```python
from build123d import *

# Parameters (mm, degrees)
SKETCH_2_R           = 9.5
EXTRUDE_1_DEPTH      = 40
SKETCH_3_W           = 6
SKETCH_3_H           = 6
EXTRUDE_2_DEPTH      = 0.1
EXTRUDE_2_DEPTH_BACK = 25
CHAMFER_1_SIZE       = 1
SKETCH_4_R           = 100
EXTRUDE_3_DEPTH      = 10
SKETCH_5_R           = 60
SKETCH_5_R_2         = 15
CUT_EXTRUDE_1_DEPTH  = 4
SKETCH_7_R           = 65
SKETCH_7_R_2         = 60
EXTRUDE_4_DEPTH      = 3.5
CHAMFER_2_SIZE       = 1
SKETCH_8_R           = 6
CUT_EXTRUDE_2_DEPTH  = 11
CHAMFER_3_SIZE       = 1
SKETCH_9_R           = 58
EXTRUDE_5_DEPTH      = 38
SKETCH_10_R          = 63
EXTRUDE_6_DEPTH      = 123
SKETCH_11_R          = 65
EXTRUDE_7_DEPTH      = 61.5
CHAMFER_4_SIZE       = 25
EXTRUDE_8_DEPTH      = 104
CUT_EXTRUDE_3_REACH  = 173
SKETCH_13_R          = 3.5
SKETCH_14_W          = 60
SKETCH_14_H          = 60
EXTRUDE_9_DEPTH      = 117
SKETCH_15_R          = 15
EXTRUDE_10_DEPTH     = 68
CHAMFER_5_SIZE       = 1
SKETCH_17_R          = 7
SKETCH_18_R          = 9
EXTRUDE_11_DEPTH     = 8
EXTRUDE_12_DEPTH     = 10
SKETCH_20_R          = 6
CUT_EXTRUDE_4_DEPTH  = 10


with BuildPart() as part:
    # Эскиз2 → Вытянуть1 (new body)
    with BuildSketch(Plane.XY):
        Circle(SKETCH_2_R)
    extrude(amount=EXTRUDE_1_DEPTH)

    # Эскиз3 → Вытянуть2 (add, two sides)
    with BuildSketch(Plane(origin=(0, 0, 0), x_dir=(-1, 0, 0), z_dir=(0, 0, -1))) as extrude_2_sk:
        with Locations((0, 9)):
            Rectangle(SKETCH_3_W, SKETCH_3_H)
    extrude(amount=EXTRUDE_2_DEPTH)
    extrude(extrude_2_sk.sketch, amount=-EXTRUDE_2_DEPTH_BACK)

    # Фаска1
    chamfer_1_edges = [part.edges().sort_by_distance(p)[0] for p in [
        (-5.556527693, -7.705517504, 0),
    ]]
    chamfer(chamfer_1_edges, length=CHAMFER_1_SIZE)

    # Эскиз4 → Вытянуть3 (add)
    with BuildSketch(Plane.XY.offset(40)):
        Circle(SKETCH_4_R)
    extrude(amount=EXTRUDE_3_DEPTH)

    # Эскиз5 → Вырез-Вытянуть1 (cut)
    with BuildSketch(Plane(origin=(0, 0, 40), x_dir=(-1, 0, 0), z_dir=(0, 0, -1))):
        Circle(SKETCH_5_R)
        Circle(SKETCH_5_R_2, mode=Mode.SUBTRACT)
    extrude(amount=-CUT_EXTRUDE_1_DEPTH, mode=Mode.SUBTRACT)

    # Эскиз7 → Вытянуть4 (add)
    with BuildSketch(Plane(origin=(0, 0, 40), x_dir=(-1, 0, 0), z_dir=(0, 0, -1))):
        with Locations(Location((0, 0, 0), (0, 0, 180))):  # turned: the seam where the file's is
            Circle(SKETCH_7_R)
        Circle(SKETCH_7_R_2, mode=Mode.SUBTRACT)
    extrude(amount=EXTRUDE_4_DEPTH)

    # Фаска2
    chamfer_2_edges = [part.edges().sort_by_distance(p)[0] for p in [
        (-65, 0, 36.5),
    ]]
    chamfer(chamfer_2_edges, length=CHAMFER_2_SIZE)

    # Эскиз8 → Вырез-Вытянуть2 (cut, through all)
    with BuildSketch(Plane(origin=(0, 0, 40), x_dir=(-1, 0, 0), z_dir=(0, 0, -1))):
        with Locations((-31.57138317, 76.220061432)):
            Circle(SKETCH_8_R)
        with Locations((31.57138317, 76.220061432)):
            Circle(SKETCH_8_R)
        with Locations((76.220061432, 31.57138317)):
            Circle(SKETCH_8_R)
        with Locations((76.220061432, -31.57138317)):
            Circle(SKETCH_8_R)
        with Locations((31.57138317, -76.220061432)):
            Circle(SKETCH_8_R)
        with Locations((-31.57138317, -76.220061432)):
            Circle(SKETCH_8_R)
        with Locations((-76.220061432, -31.57138317)):
            Circle(SKETCH_8_R)
        with Locations((-76.220061432, 31.57138317)):
            Circle(SKETCH_8_R)
    extrude(amount=-CUT_EXTRUDE_2_DEPTH, mode=Mode.SUBTRACT)

    # Фаска3
    chamfer_3_edges = [part.edges().sort_by_distance(p)[0] for p in [
        (15, 0, 40),
    ]]
    chamfer(chamfer_3_edges, length=CHAMFER_3_SIZE)

    # Эскиз9 → Вытянуть5 (add)
    with BuildSketch(Plane.XY.offset(50)):
        Circle(SKETCH_9_R)
    extrude(amount=EXTRUDE_5_DEPTH)

    # Эскиз10 → Вытянуть6 (add)
    with BuildSketch(Plane.XY.offset(88)):
        Circle(SKETCH_10_R)
    extrude(amount=EXTRUDE_6_DEPTH)

    # Эскиз11 → Вытянуть7 (add)
    with BuildSketch(Plane.XY.offset(211)):
        Circle(SKETCH_11_R)
    extrude(amount=EXTRUDE_7_DEPTH)

    # Фаска4
    chamfer_4_edges = [part.edges().sort_by_distance(p)[0] for p in [
        (-65, 0, 272.5),
    ]]
    chamfer(chamfer_4_edges, length=CHAMFER_4_SIZE)

    # Эскиз12 → Вытянуть8 (add)
    with BuildSketch(Plane(origin=(0, 0, 88), x_dir=(-1, 0, 0), z_dir=(0, 0, -1))):
        Polygon((-45.686291501, -71), (-63, -71), (-63, -63), (-49, -63), (-34.844951906, -48.844951906), (-27.837639703, -53.151348202), align=None)
        Polygon((45.686291501, -71), (63, -71), (63, -63), (49, -63), (34.844951906, -48.844951906), (27.837639703, -53.151348202), align=None)
    extrude(amount=-EXTRUDE_8_DEPTH)

    # Эскиз13 → Вырез-Вытянуть3 (cut, up to next)
    with BuildSketch(Plane.XZ.offset(71), mode=Mode.PRIVATE) as cut_extrude_3_sk1:
        with Locations(Location((-56, 95, 0), (0, 0, 270))):  # turned: the seam where the file's is
            Circle(SKETCH_13_R)
    cut_extrude_3_tool1 = extrude(cut_extrude_3_sk1.sketch, amount=-CUT_EXTRUDE_3_REACH, mode=Mode.PRIVATE) & part.part
    add(cut_extrude_3_tool1.solids().sort_by_distance((-56, -71, 95))[0], mode=Mode.SUBTRACT)
    # Эскиз13 → Вырез-Вытянуть3 (cut, up to next)
    with BuildSketch(Plane.XZ.offset(71), mode=Mode.PRIVATE) as cut_extrude_3_sk2:
        with Locations(Location((56, 95, 0), (0, 0, 270))):  # turned: the seam where the file's is
            Circle(SKETCH_13_R)
    cut_extrude_3_tool2 = extrude(cut_extrude_3_sk2.sketch, amount=-CUT_EXTRUDE_3_REACH, mode=Mode.PRIVATE) & part.part
    add(cut_extrude_3_tool2.solids().sort_by_distance((56, -71, 95))[0], mode=Mode.SUBTRACT)
    # Эскиз13 → Вырез-Вытянуть3 (cut, up to next)
    with BuildSketch(Plane.XZ.offset(71), mode=Mode.PRIVATE) as cut_extrude_3_sk3:
        with Locations(Location((-56, 185, 0), (0, 0, 270))):  # turned: the seam where the file's is
            Circle(SKETCH_13_R)
    cut_extrude_3_tool3 = extrude(cut_extrude_3_sk3.sketch, amount=-CUT_EXTRUDE_3_REACH, mode=Mode.PRIVATE) & part.part
    add(cut_extrude_3_tool3.solids().sort_by_distance((-56, -71, 185))[0], mode=Mode.SUBTRACT)
    # Эскиз13 → Вырез-Вытянуть3 (cut, up to next)
    with BuildSketch(Plane.XZ.offset(71), mode=Mode.PRIVATE) as cut_extrude_3_sk4:
        with Locations(Location((56, 185, 0), (0, 0, 270))):  # turned: the seam where the file's is
            Circle(SKETCH_13_R)
    cut_extrude_3_tool4 = extrude(cut_extrude_3_sk4.sketch, amount=-CUT_EXTRUDE_3_REACH, mode=Mode.PRIVATE) & part.part
    add(cut_extrude_3_tool4.solids().sort_by_distance((56, -71, 185))[0], mode=Mode.SUBTRACT)

    # Эскиз14 → Вытянуть9 (add)
    with BuildSketch(Plane(origin=(0, 0, 0), x_dir=(1, 0, 0), z_dir=(0, 1, 0))):
        with Locations((0, -119)):
            Rectangle(SKETCH_14_W, SKETCH_14_H)
    extrude(amount=EXTRUDE_9_DEPTH)

    # Эскиз15 → Вытянуть10 (add)
    with BuildSketch(Plane(origin=(0, 0, 0), x_dir=(1, 0, 0), z_dir=(0, 1, 0))):
        with Locations(Location((0, -165, 0), (0, 0, 90))):  # turned: the seam where the file's is
            Circle(SKETCH_15_R)
    extrude(amount=EXTRUDE_10_DEPTH)

    # Фаска5
    chamfer_5_edges = [part.edges().sort_by_distance(p)[0] for p in [
        (0, 68, 180),
    ]]
    chamfer(chamfer_5_edges, length=CHAMFER_5_SIZE)

    # По траектории1: sweep along a path in Эскиз16
    with BuildLine(Plane.XY.offset(165)) as sweep_1_path:
        CenterArc((0, 86), 18, 0, 360)
    # Эскиз17 → По траектории1 (sweep)
    with BuildSketch(Plane(origin=(0, 0, 0), x_dir=(0, 0, -1), z_dir=(1, 0, 0))):
        with Locations((-165, 104)):
            Circle(SKETCH_17_R)
    sweep(path=sweep_1_path.line)

    # Эскиз18 → Вытянуть11 (add)
    with BuildSketch(Plane.ZY.offset(30)):
        with Locations(Location((119, 87, 0), (0, 0, 180))):  # turned: the seam where the file's is
            Circle(SKETCH_18_R)
    extrude(amount=EXTRUDE_11_DEPTH)

    # Эскиз19 → Вытянуть12 (add)
    with BuildSketch(Plane.ZY.offset(38)):
        Polygon((119, 102.588457268), (105.5, 94.794228634), (105.5, 79.205771366), (119, 71.411542732), (132.5, 79.205771366), (132.5, 94.794228634), align=None)
    extrude(amount=EXTRUDE_12_DEPTH)

    # Эскиз20 → Вырез-Вытянуть4 (cut)
    with BuildSketch(Plane.ZY.offset(48)):
        with Locations((119, 87)):
            Circle(SKETCH_20_R)
    extrude(amount=-CUT_EXTRUDE_4_DEPTH, mode=Mode.SUBTRACT)


solid = part.part
```
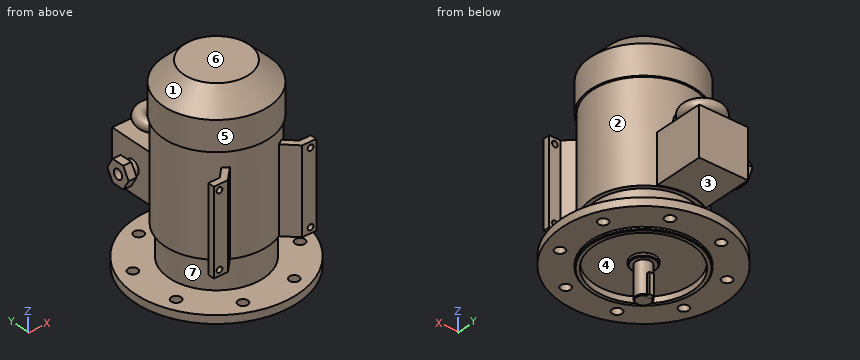
Geometry: final body of the model. Coordinates: model frame, mm. Face numbers are marked on the shaded views. A direction names the side the tool comes from. Coordinates: 2 decimals unless noted, no trailing zeros. Order: outer loops, then holes, each group sorted by start corner. A loop starts at its lowest first (then second) coordinate and runs counter-clockwise, first axis right, second up. Notation, with made-up numbers: (82.25, -29.5) -> (110.25, -29.5) arc R14 ccw to (110.25, -18.5) -> close; hole circle Ø1 at (13.25, -11.75). An arc over 180 degrees is marked (long way). Write each question's results on one line, items separated by ' | '. Start each with the question number.
1) Mould query, pull axis Y, two halves, no side actions, for the marked faces 1, 2 and 3. Classes: released by +Y, released by -Y, zero draft, split by the parting line, or undercut.
2) First-contact query: pin 1 (3 mm diameter, centred on y = 46, z = 159.5, fed in from +X); pin 2 (7 mm diameter, centred on x = -57, z = 152, fed in from +Y); pin 3 (2 mm diameter, centred on y = 33.5, z = 145.5, fed in from -X). Flat tips, straight axial feed; report the tip coordinate or a pass-through.
3) Material intervals for line 1 along Y through (x, z) = (0, 41); line 2 along X through (y, z) = (-65, 185); line 3 along X through (y, z) = (-65.75, 95), sorted ascending.
4) Cut plane A-A, the plane z = 165. Output: boundary loops of the cut face in (x, y).
5) Cut plane B-B, the plane z = 95. Output: boundary loops of the cut face in (x, y), and give its area (3 significant figures).
6) Cut plane C-C, the plane z = 31. Output: boundary loops of the cut face in (x, y).
7) Set-up query: the marked faces 4, 5, 6 and 7. Return all of +Z, -Z, +X, -X, +Y, -Y with unobstructed straight access to the full face (end or side cutting, diameter ignored); none if empty.
Checks:
1) face 1: split by the parting line | face 2: undercut | face 3: zero draft
2) pin 1: x = 44.6 | pin 2: y = 33.27 | pin 3: x = -53.97
3) line 1: -100 to -60, -15 to 15, 60 to 100 | line 2: -63 to -59.5, -52.5 to -39.69, 39.69 to 52.5, 59.5 to 63 | line 3: -63 to -59.5, -52.5 to -40.44, 40.44 to 52.5, 59.5 to 63
4) outline: (-63, -71) -> (-45.69, -71) -> (-30.06, -55.37) arc R63 ccw to (30.06, -55.37) -> (45.69, -71) -> (63, -71) -> (63, -63) -> (49, -63) -> (36.99, -50.99) arc R63 ccw to (15, 61.19) -> (15, 66) arc R25 ccw (long way) to (-15, 66) -> (-15, 61.19) arc R63 ccw to (-36.99, -50.99) -> (-49, -63) -> (-63, -63) -> close; hole circle Ø22 at (0, 86)
5) outline: (-63, -71) -> (-59.5, -71) -> (-59.5, -63) -> (-63, -63) -> close; (-52.5, -71) -> (-45.69, -71) -> (-30.06, -55.37) arc R63 ccw to (30.06, -55.37) -> (45.69, -71) -> (52.5, -71) -> (52.5, -63) -> (49, -63) -> (36.99, -50.99) arc R63 ccw to (30, 55.4) -> (30, 117) -> (-30, 117) -> (-30, 55.4) arc R63 ccw to (-36.99, -50.99) -> (-49, -63) -> (-52.5, -63) -> close; (59.5, -71) -> (63, -71) -> (63, -63) -> (59.5, -63) -> close | area: 16,300 mm^2
6) outline: circle Ø19 at (0, 0)
7) face 4: -Z | face 5: +Z | face 6: +Z, +X, -X, +Y, -Y | face 7: none
